Could you check a few things on this model? Use its own coordinates, in mm. Face numbers are marked on the shaded views. A direction names the side the tool comes from. Give positions to 0.01 mm unless a question says otherwise; leave off trailing zeros. Loops run counter-clockwise (first coordinate to the right, second up) from the corner with the lowest first, then second, coordinate; pieces in that order, holes last. Notation, with made-up numbers: M -25,-20 L 29,-20 A19 ccw 29,14 Z; hole C 71.5,34.25 d7. An arc over 180 degrees is marked long. Use a Markdown table: item, result. Add a question column.
1) If I drill on line 1 along X through (y, z) = (27.6, 0); line 2 along Y through (x, z) = (-1, -25); line 3 along X through (y, z) = (28, 16), over which ranges is the centre line in solid material (lowest first)? Write a range as [from, to].
2) Suppose I cut it at D-D on x = 0. Count the separate pieces of the cut face and the enclosed holes in it, and give its area (3 significant figures).
3) Suppose I cut it at B-B on z = -16.5. List the corners of the cut face in (x, y) for me.
4) Will these pins go through, and if not, where does the flat tip stop? pin 1 Ø12 at (x, y) = (20.5, 26) entering from -Z; pin 2 Ø1.8 at (x, z) = (-13, -0.5) entering from +Y; pin 3 Ø12 at (y, z) = (21, 23) entering from +X.
5) Suppose I cut it at A-A on y = 7.5. List the corners of the cut face in (x, z) for me (3 decimals).
6) Suppose I cut it at C-C on x = -23. List the corners of the cut face in (y, z) for me, and give its area (3 significant figures).
7) We'd pull the mould along Z, two halves only. Please class the marked faces 1, 2 and 3: +Z half, -Z half, draft (parallel to the pull), parting line (faces both ways), or undercut.
8) Which directions (+Z, -Z, +X, -X, +Y, -Y) give clear straight access to the entire face, cutting with the end or side of a thin tool? Please do the marked faces 4, 5 and 6.
```python
from build123d import *

# Parameters (mm, degrees)
SKETCH1_R           = 30
BOSS_EXTRUDE1_DEPTH = 30.5
SKETCH4_R           = 5
CUT_EXTRUDE2_DEPTH  = 30.5
CUT_EXTRUDE3_DEPTH  = 25
CIRPATTERN1_COUNT   = 6
CUT_EXTRUDE4_START  = -25.5
SKETCH13_R          = 26
CUT_EXTRUDE4_DEPTH  = 25.5
CHAMFER1_SIZE       = 2
BOSS_EXTRUDE2_DEPTH = 5.5
SKETCH17_R          = 1.6
CUT_EXTRUDE5_DEPTH  = 5.5
CIRPATTERN2_COUNT   = 6
SKETCH19_R          = 1.55
CUT_EXTRUDE6_DEPTH  = 5
SKETCH20_R          = 2
CUT_EXTRUDE7_DEPTH  = 4
CIRPATTERN3_COUNT   = 4
SKETCH21_R          = 1.5
CUT_EXTRUDE8_DEPTH  = 5
SKETCH22_R          = 1.5
CUT_EXTRUDE9_DEPTH  = 5
SKETCH23_R          = 3
CUT_EXTRUDE10_DEPTH = 3
CIRPATTERN5_COUNT   = 2


with BuildPart() as part:
    # Sketch1 → Boss-Extrude1 (new body)
    with BuildSketch(Plane(origin=(0, 0, 0), x_dir=(1, 0, 0), z_dir=(0, 1, 0))):
        with Locations(Location((0, 0, 0), (0, 0, 90))):
            Circle(SKETCH1_R)
    extrude(amount=BOSS_EXTRUDE1_DEPTH)

    # Sketch4 → Cut-Extrude2 (cut)
    with BuildSketch(Plane(origin=(0, 30.5, 0), x_dir=(1, 0, 0), z_dir=(0, 1, 0))):
        with Locations(Location((0, 0, 0), (0, 0, 270))):
            Circle(SKETCH4_R)
    extrude(amount=-CUT_EXTRUDE2_DEPTH, mode=Mode.SUBTRACT)

    # Sketch5 → Cut-Extrude3 (cut)
    with BuildSketch(Plane(origin=(0, 30.5, 0), x_dir=(1, 0, 0), z_dir=(0, 1, 0))):
        with BuildLine():
            Line((-12.825755375, 35.238473279), (-8.892523726, 24.43200814))
            ThreePointArc((-8.892523726, 24.43200814), (0, 26), (8.892523726, 24.43200814))
            Line((8.892523726, 24.43200814), (12.825755375, 35.238473279))
            ThreePointArc((12.825755375, 35.238473279), (0, 37.5), (-12.825755375, 35.238473279))
        make_face()
    cut_extrude3 = extrude(amount=-CUT_EXTRUDE3_DEPTH, mode=Mode.SUBTRACT)

    # CirPattern1: Cut-Extrude3 ×6 about axis
    cirpattern1_axis = Axis((0, 0, 0), (0, 1, 0))
    for i in range(1, CIRPATTERN1_COUNT):
        add(cut_extrude3.rotate(cirpattern1_axis, i * 360 / CIRPATTERN1_COUNT), mode=Mode.SUBTRACT)

    # Sketch13 → Cut-Extrude4 (cut)
    with BuildSketch(Plane.XZ.offset(CUT_EXTRUDE4_START)):
        with Locations(Location((0, 0, 0), (0, 0, 270))):
            Circle(SKETCH13_R)
    extrude(amount=CUT_EXTRUDE4_DEPTH, mode=Mode.SUBTRACT)

    # Chamfer1
    chamfer1_edges = [part.edges().sort_by_distance(p)[0] for p in [
        (-15, 30.5, -25.980762114),
        (-30, 30.5, 0),
        (-15, 30.5, 25.980762114),
        (15, 30.5, 25.980762114),
        (30, 30.5, 0),
        (15, 30.5, -25.980762114),
    ]]
    chamfer(chamfer1_edges, length=CHAMFER1_SIZE)

    # Sketch15 → Boss-Extrude2 (add)
    with BuildSketch(Plane.XZ):
        with BuildLine():
            Line((-3.391631546, 27.864196424), (3.391631546, 27.864196424))
            ThreePointArc((3.391631546, 27.864196424), (0, 23.5), (-3.391631546, 27.864196424))
        make_face()
    boss_extrude2 = extrude(amount=-BOSS_EXTRUDE2_DEPTH)

    # Sketch17 → Cut-Extrude5 (cut)
    with BuildSketch(Plane.XZ):
        with Locations(Location((0, 27, 0), (0, 0, 270))):
            Circle(SKETCH17_R)
    cut_extrude5 = extrude(amount=-CUT_EXTRUDE5_DEPTH, mode=Mode.SUBTRACT)

    # CirPattern2: Boss-Extrude2, Cut-Extrude5 ×6 about axis
    cirpattern2_axis = Axis((0, 0, 0), (0, 1, 0))
    add([boss_extrude2.rotate(cirpattern2_axis, i * 360 / CIRPATTERN2_COUNT) for i in range(1, CIRPATTERN2_COUNT)])
    add([cut_extrude5.rotate(cirpattern2_axis, i * 360 / CIRPATTERN2_COUNT) for i in range(1, CIRPATTERN2_COUNT)], mode=Mode.SUBTRACT)

    # Sketch19 → Cut-Extrude6 (cut)
    with BuildSketch(Plane(origin=(0, 30.5, 0), x_dir=(1, 0, 0), z_dir=(0, 1, 0))):
        with Locations(Location((-16.5, 16.5, 0), (0, 0, 270))):
            Circle(SKETCH19_R)
    cut_extrude6 = extrude(amount=-CUT_EXTRUDE6_DEPTH, mode=Mode.SUBTRACT)

    # Sketch20 → Cut-Extrude7 (cut)
    with BuildSketch(Plane.XZ.offset(-25.5)):
        with Locations(Location((-16.5, -16.5, 0), (0, 0, 270))):
            Circle(SKETCH20_R)
    cut_extrude7 = extrude(amount=-CUT_EXTRUDE7_DEPTH, mode=Mode.SUBTRACT)

    # CirPattern3: Cut-Extrude6, Cut-Extrude7 ×4 about axis
    cirpattern3_axis = Axis((0, 0, 0), (0, 1, 0))
    add([cut_extrude6.rotate(cirpattern3_axis, i * 360 / CIRPATTERN3_COUNT) for i in range(1, CIRPATTERN3_COUNT)], mode=Mode.SUBTRACT)
    add([cut_extrude7.rotate(cirpattern3_axis, i * 360 / CIRPATTERN3_COUNT) for i in range(1, CIRPATTERN3_COUNT)], mode=Mode.SUBTRACT)

    # Sketch21 → Cut-Extrude8 (cut)
    with BuildSketch(Plane(origin=(0, 30.5, 0), x_dir=(1, 0, 0), z_dir=(0, 1, 0))):
        with Locations(Location((0, 9.5, 0), (0, 0, 270))):
            Circle(SKETCH21_R)
    cut_extrude8 = extrude(amount=-CUT_EXTRUDE8_DEPTH, mode=Mode.SUBTRACT)

    # Sketch22 → Cut-Extrude9 (cut)
    with BuildSketch(Plane(origin=(0, 30.5, 0), x_dir=(1, 0, 0), z_dir=(0, 1, 0))):
        with Locations(Location((-12.5, 0, 0), (0, 0, 270))):
            Circle(SKETCH22_R)
    cut_extrude9 = extrude(amount=-CUT_EXTRUDE9_DEPTH, mode=Mode.SUBTRACT)

    # Sketch23 → Cut-Extrude10 (cut)
    with BuildSketch(Plane(origin=(0, 30.5, 0), x_dir=(1, 0, 0), z_dir=(0, 1, 0))):
        with Locations(Location((0, 9.5, 0), (0, 0, 270))):
            Circle(SKETCH23_R)
        with Locations(Location((-12.5, 0, 0), (0, 0, 270))):
            Circle(SKETCH23_R)
    cut_extrude10 = extrude(amount=-CUT_EXTRUDE10_DEPTH, mode=Mode.SUBTRACT)

    # CirPattern5: Cut-Extrude8, Cut-Extrude9, Cut-Extrude10 ×2 about axis
    cirpattern5_axis = Axis((0, 0, 0), (0, 1, 0))
    add([cut_extrude8.rotate(cirpattern5_axis, i * 360 / CIRPATTERN5_COUNT) for i in range(1, CIRPATTERN5_COUNT)], mode=Mode.SUBTRACT)
    add([cut_extrude9.rotate(cirpattern5_axis, i * 360 / CIRPATTERN5_COUNT) for i in range(1, CIRPATTERN5_COUNT)], mode=Mode.SUBTRACT)
    add([cut_extrude10.rotate(cirpattern5_axis, i * 360 / CIRPATTERN5_COUNT) for i in range(1, CIRPATTERN5_COUNT)], mode=Mode.SUBTRACT)


solid = part.part
```
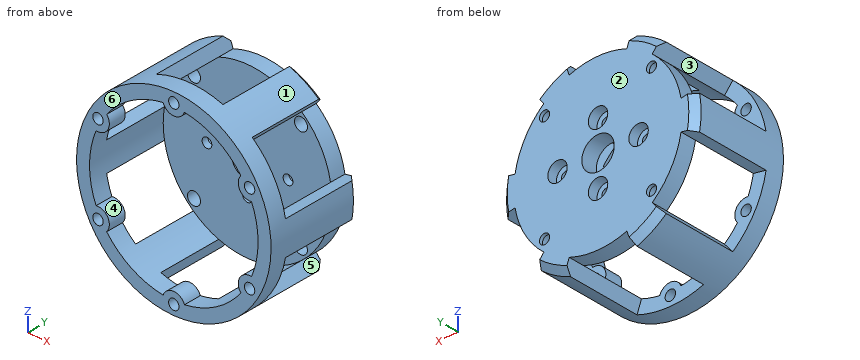
Answer block:
| question | item | result |
|---|---|---|
| 1 | line 1 | x = [-30, -15.5], [-9.5, -5], [5, 9.5], [15.5, 30] |
| 1 | line 2 | y = [0, 5.5], [25.5, 30.5] |
| 1 | line 3 | x = [-20.49, -18.44], [-14.56, 14.56], [18.44, 20.49] |
| 2 | separate pieces | 8 |
| 2 | enclosed holes | 0 |
| 2 | area | 198 mm^2 |
| 3 | outline | M -25.05,0 L -20.09,0 L -20.09,5.5 L -25.05,5.5 Z; M -20.09,25.5 L -18.5,25.5 L -18.5,29.5 L -18.05,29.5 L -18.05,30.5 L -20.09,30.5 Z; M -14.95,29.5 L -14.5,29.5 L -14.5,25.5 L 14.5,25.5 L 14.5,29.5 L 14.95,29.5 L 14.95,30.5 L -14.95,30.5 Z; M 18.05,29.5 L 18.5,29.5 L 18.5,25.5 L 20.09,25.5 L 20.09,30.5 L 18.05,30.5 Z; M 20.09,0 L 25.05,0 L 25.05,5.5 L 20.09,5.5 Z |
| 4 | pin 1 | stops at z = -26.26 |
| 4 | pin 2 | stops at y = 27.5 |
| 4 | pin 3 | stops at x = 19.28 |
| 5 | outline | M -29.544,-5.209 L -25.605,-4.515 A26 cw -25.605,4.515 L -29.544,5.209 A30 ccw Z; M -19.284,-22.981 A30 ccw -10.261,-28.191 L -8.893,-24.432 A26 cw -16.712,-19.917 Z; M -19.284,22.981 L -16.712,19.917 A26 cw -8.893,24.432 L -10.261,28.191 A30 ccw Z; M 8.893,-24.432 L 10.261,-28.191 A30 ccw 19.284,-22.981 L 16.712,-19.917 A26 cw Z; M 8.893,24.432 A26 cw 16.712,19.917 L 19.284,22.981 A30 ccw 10.261,28.191 Z; M 25.605,-4.515 L 29.544,-5.209 A30 ccw 29.544,5.209 L 25.605,4.515 A26 cw Z |
| 6 | outline | M 0,-19.26 L 5.5,-19.26 L 5.5,-15.05 L 0,-15.05 Z; M 0,-11.95 L 5.5,-11.95 L 5.5,-10.02 L 0,-10.02 Z; M 0,10.02 L 5.5,10.02 L 5.5,11.95 L 0,11.95 Z; M 0,15.05 L 5.5,15.05 L 5.5,19.26 L 0,19.26 Z; M 25.5,-12.12 L 30.5,-12.12 L 30.5,12.12 L 25.5,12.12 Z |
| 6 | area | 189 mm^2 |
| 7 | face 1 | parting line |
| 7 | face 2 | draft |
| 7 | face 3 | undercut |
| 8 | face 4 | -Y |
| 8 | face 5 | +X, +Y |
| 8 | face 6 | +Z, -Z, +X, -X, -Y |
